Job drawing, mm, ordinate dimensions from the low corner. One solid piece. Give positions to 0.01 mm unless a question says otherwise; leave off trailing zeros. Order: outer loops, then holes, each group sorted by start corner. A loop starts at its lowest first (then second) coordinate and runs counter-clockwise, first axis right, second up. Notation, with made-up numbers: (0, -31) -> (37, -31) arc R14 cw to (37, -6) -> close; hole circle Ø7 at (-23.5, -38.75). An arc over 180 degrees is marked (long way). Write item = value, one per line. Start each with the question number.
(1) Saw through at D-D, the plane z = 21. List the corners of the cut face in (x, y), then the cut area to 3 significant figures.
(2) Probe line 1 along X through (y, z) = (0.1, 4); line 2 along X through (y, z) = (0.35, 19); line 3 along X through (y, z) = (0.2, 13.5). List the from-to ranges inside material, lowest first. Write a range as from..to.
(3) Saw through at B-B, the plane z = 6.5. List the corners of the cut face in (x, y).
(4) Saw through at C-C, the plane y = 0.1. List the corners of the cut face in (x, z).
(5) Saw through at A-A, the plane x = 16. List the corners of the cut face in (y, z), then the cut area to 3 significant figures.
(6) Flat gauge pin, fed straight in: pin 1 (8 mm diameter, centred on x = 15, z = 21.5, fed in from -Y). Where does the tip first touch, or does it go through?
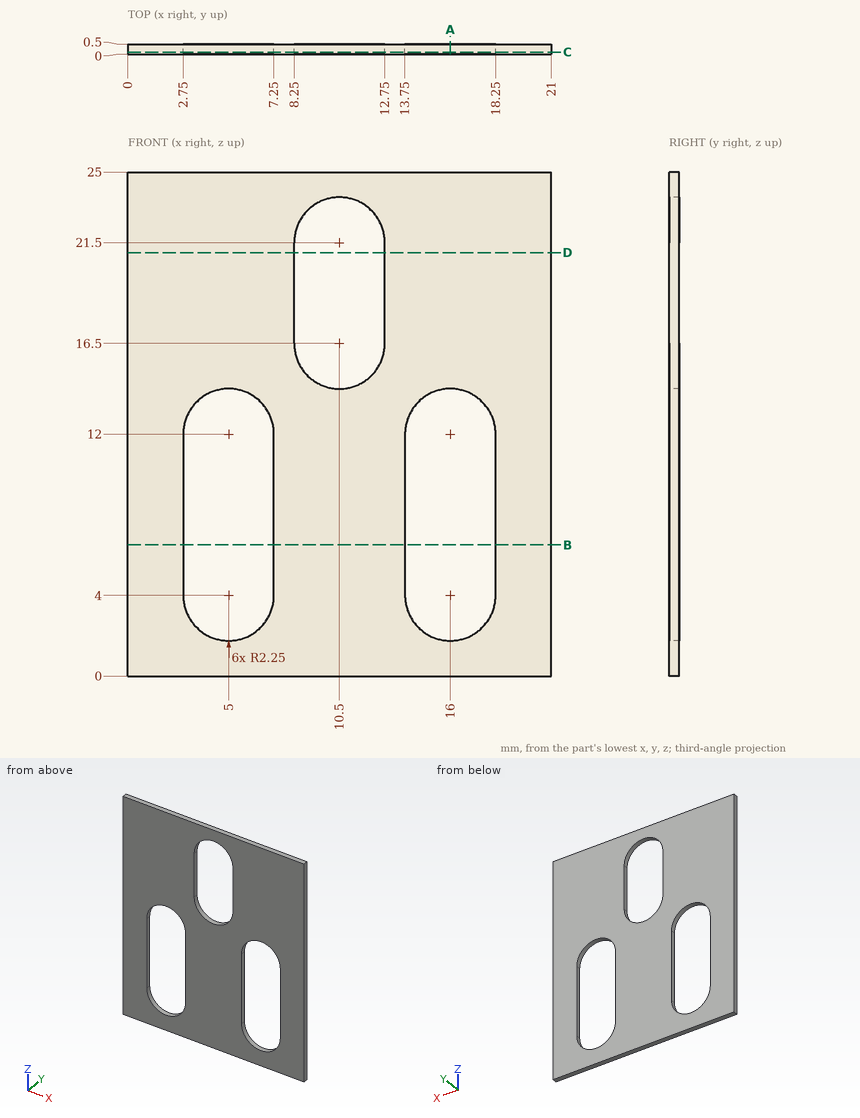
Results list:
q1.outline = (0, 0) -> (8.25, 0) -> (8.25, 0.5) -> (0, 0.5) -> close; (12.75, 0) -> (21, 0) -> (21, 0.5) -> (12.75, 0.5) -> close
q1.area = 8.25 mm^2
q2.line_1 = 0..2.75, 7.25..13.75, 18.25..21
q2.line_2 = 0..8.25, 12.75..21
q2.line_3 = 0..3.32, 6.68..14.32, 17.68..21
q3.outline = (0, 0) -> (2.75, 0) -> (2.75, 0.5) -> (0, 0.5) -> close; (7.25, 0) -> (13.75, 0) -> (13.75, 0.5) -> (7.25, 0.5) -> close; (18.25, 0) -> (21, 0) -> (21, 0.5) -> (18.25, 0.5) -> close
q4.outline = (0, 0) -> (21, 0) -> (21, 25) -> (0, 25) -> close; hole (2.75, 4) arc R2.25 ccw to (7.25, 4) -> (7.25, 12) arc R2.25 ccw to (2.75, 12) -> close; hole (8.25, 16.5) arc R2.25 ccw to (12.75, 16.5) -> (12.75, 21.5) arc R2.25 ccw to (8.25, 21.5) -> close; hole (13.75, 4) arc R2.25 ccw to (18.25, 4) -> (18.25, 12) arc R2.25 ccw to (13.75, 12) -> close
q5.outline = (0, 0) -> (0.5, 0) -> (0.5, 1.75) -> (0, 1.75) -> close; (0, 14.25) -> (0.5, 14.25) -> (0.5, 25) -> (0, 25) -> close
q5.area = 6.25 mm^2
q6.pin_1 = 0
